```python
from build123d import *

# Parameters (mm, degrees)
BOSS_EXTRUDE1_DEPTH = 25.4
FILLET1_R           = 8


with BuildPart() as part:
    # Sketch1 → Boss-Extrude1 (new body)
    with BuildSketch(Plane.XY):
        Polygon((7, -61.2), (-5, -27.8), (-5, 27.8), (7.829493088, 74.2), (35, 74.2), (41, 48.7), (41, -48.7), (48.216878365, -61.2), (32, -61.2), (32, -71.2), (145, -71.2), (145, -61.2), (128.783121635, -61.2), (136, -48.7), (136, 48.7), (142, 74.2), (169.170506912, 74.2), (182, 27.8), (182, -27.8), (170, -61.2), (175.646616425, -63.228724464), (190, -23.278473513), (190, 28.88562364), (174.152706997, 86.2), (128, 86.2), (128, -46.556406461), (119.545517328, -61.2), (57.454482672, -61.2), (49, -46.556406461), (49, 86.2), (2.847293003, 86.2), (-13, 28.88562364), (-13, -23.278473513), (1.353383575, -63.228724464), align=None)
    extrude(amount=-BOSS_EXTRUDE1_DEPTH)

    # Fillet1
    fillet1_edges = [part.edges().sort_by_distance(p)[0] for p in [
        (49, 86.2, -12.7),
        (128, 86.2, -12.7),
    ]]
    fillet(fillet1_edges, radius=FILLET1_R)


solid = part.part
```
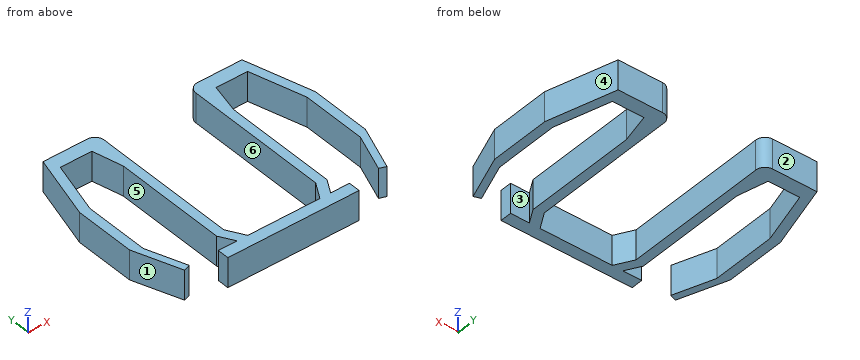
Work out the finished part from the listing and answer in its coordinate system (mm). Face numbers are marked on the shaded views. A direction names the side the tool comes from. Coordinates: 2 decimals unless noted, no trailing zeros. Write each loop counter-clockwise with the first axis right and the second up, starting at its lowest first coordinate (ties: lowest second). Pieces come first, ordered by that corner, then holes. Notation, with made-up numbers: (-39.75, 69) - (-33.75, 69) arc R19 ccw to (-33.75, 100) - close; hole circle Ø6 at (74, 8). An arc over 180 degrees is marked (long way). Answer as a JSON object with one key per item and string values.
Q1. Given pin 1 Ø1 at (y, z) = (-34, -5.5) entering from +X; pin 2 Ø11 at (y, z) = (-68, -11) entering from +X; pin 3 Ø10 at (y, z) = (49, -19) entering from -X, each flat-ended and moving along its own axis, determine where each tip first touches the part or whether it passes through.
Results list:
{"pin 1": "stops at x = 186.33", "pin 2": "stops at x = 175.91", "pin 3": "stops at x = -8.82"}
Q2. Find section C-C (y = -38.5). Write down the section's boundary in (x, z).
Results list:
{"outline": "(-7.53, -25.4) - (-1.16, -25.4) - (-1.16, 0) - (-7.53, 0) - close; (41, -25.4) - (49, -25.4) - (49, 0) - (41, 0) - close; (128, -25.4) - (136, -25.4) - (136, 0) - (128, 0) - close; (178.16, -25.4) - (184.53, -25.4) - (184.53, 0) - (178.16, 0) - close"}
Q3. For a pull along X with two mould halves and no side action, classify the marked faces 1, 2 and 3 as pulls with the +X half, pulls with the -X half, needs draft (parallel to the pull), parting line crosses it, or undercut.
Results list:
{"face 1": "pulls with the -X half", "face 2": "needs draft", "face 3": "undercut"}
Q4. Find section B-B (x = 15). Write down the section's boundary in (y, z), plus the area to 3 significant figures.
Results list:
{"outline": "(74.2, -25.4) - (86.2, -25.4) - (86.2, 0) - (74.2, 0) - close", "area": "305 mm^2"}
Q5. Consider L1, parallel to X at y = -1, z = -14.5; L2, parallel to X at y = 40, z = -9; L3, parallel to Y at x = 23, z = -5.75. Determine where each line is inside the solid, lowest interval first. Write a range as from..to.
Results list:
{"L1": "x = -13..-5, 41..49, 128..136, 182..190", "L2": "x = -9.93..-1.63, 41..49, 128..136, 178.63..186.93", "L3": "y = 74.2..86.2"}
Q6. Find section A-A (y = 57). Write down the section's boundary in (x, z).
Results list:
{"outline": "(-5.23, -25.4) - (3.07, -25.4) - (3.07, 0) - (-5.23, 0) - close; (39.05, -25.4) - (49, -25.4) - (49, 0) - (39.05, 0) - close; (128, -25.4) - (137.95, -25.4) - (137.95, 0) - (128, 0) - close; (173.93, -25.4) - (182.23, -25.4) - (182.23, 0) - (173.93, 0) - close"}
Q7. Find section D-D (x = 75.5). Write down the section's boundary in (y, z), plus the area to 3 significant figures.
Results list:
{"outline": "(-71.2, -25.4) - (-61.2, -25.4) - (-61.2, 0) - (-71.2, 0) - close", "area": "254 mm^2"}
Q8. Which of the six approach directions +Z, -Z, +X, -X, +Y, -Y give full straight-line access (tool end or side, diameter ignored) to the marked faces 4, 5 and 6?
Results list:
{"face 4": "+Z, -Z, +X, +Y", "face 5": "+Z, -Z", "face 6": "+Z, -Z, +Y"}
